```python
from build123d import *

# Parameters (mm, degrees)
SKETCH1_W           = 279.4
SKETCH1_H           = 275.43125
SKETCH1_R           = 6.35
SKETCH1_R_2         = 12.7
BOSS_EXTRUDE1_DEPTH = 2.54


with BuildPart() as part:
    # Sketch1 → Boss-Extrude1 (new body)
    with BuildSketch(Plane.XY):
        Rectangle(SKETCH1_W, SKETCH1_H)
        with Locations((-127, 125.015625)):
            Circle(SKETCH1_R, mode=Mode.SUBTRACT)
        with Locations(Location((-127, -125.015625, 0), (0, 0, 180))):
            Circle(SKETCH1_R, mode=Mode.SUBTRACT)
        with Locations((127, -125.015625)):
            Circle(SKETCH1_R, mode=Mode.SUBTRACT)
        with Locations(Location((127, 125.015625, 0), (0, 0, 180))):
            Circle(SKETCH1_R, mode=Mode.SUBTRACT)
        with Locations((0, 20.240625)):
            Circle(SKETCH1_R_2, mode=Mode.SUBTRACT)
    extrude(amount=BOSS_EXTRUDE1_DEPTH)


solid = part.part
```
Verification items for the finished model (mm, model axes). Round coordinates to 2 decimals unless told otherwise and drop trailing zeros. Order: outer loops, then holes, each group sorted by start corner. A loop starts at its lowest first (then second) coordinate and runs counter-clockwise, first axis right, second up. Notation, with made-up numbers: (-18, -33) - (28, -33) arc R14 cw to (28, -27) - close; hole circle Ø9 at (67.25, -39). An arc over 180 degrees is marked (long way). Use CSV: the item, a comma, the result in double quotes.
(1) Section check A-A on x = 0. Record the boundary of the cut face in (y, z).
Entries:
outline,"(-137.72, 0) - (7.54, 0) - (7.54, 2.54) - (-137.72, 2.54) - close; (32.94, 0) - (137.72, 0) - (137.72, 2.54) - (32.94, 2.54) - close"
(2) Mould release check, pull along Y, two halves, no side actions. Record for faces 1 (the face through (-2, 2, 2.54)), 2 (the face through (-2.75, 7.84, 1.25)): released by +Y, released by -Y, zero draft, split by the parting line, or undercut.
Entries:
face 1,"zero draft"
face 2,"undercut"
(3) Section check B-B on x = -127. Record the boundary of the cut face in (y, z), and give its area (3 significant figures).
Entries:
outline,"(-137.72, 0) - (-131.37, 0) - (-131.37, 2.54) - (-137.72, 2.54) - close; (-118.67, 0) - (118.67, 0) - (118.67, 2.54) - (-118.67, 2.54) - close; (131.37, 0) - (137.72, 0) - (137.72, 2.54) - (131.37, 2.54) - close"
area,"635 mm^2"
(4) Thickness scan on probe 1 along Y at (x, z) = (127, 0.9); probe 2 along Y at (x, z) = (0, 0.7); probe 3 along X at (y, z) = (17, 0.3). Record the ranges inside material, lowest first. Write a range as from..to.
Entries:
probe 1,"-137.72..-131.37, -118.67..118.67, 131.37..137.72"
probe 2,"-137.72..7.54, 32.94..137.72"
probe 3,"-139.7..-12.28, 12.28..139.7"
